Part model, mm, in its own coordinate system. Face numbers are marked on the shaded views. A direction names the side the tool comes from. Round coordinates to 2 decimals unless told otherwise and drop trailing zeros. Loops run counter-clockwise (first coordinate to the right, second up) from the corner with the lowest first, then second, coordinate; pieces in that order, holes last. Notation, with made-up numbers: (50.5, 60) - (78.5, 60) arc R15 ccw to (78.5, 79) - close; hole circle Ø3 at (12, 45.5). An arc over 180 degrees is marked (long way). Put each result on its own line as item: value.
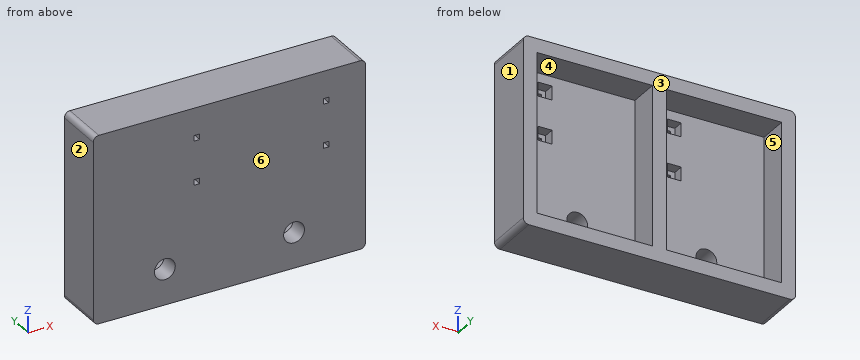
from build123d import *

# Parameters (mm, degrees)
SKETCH1_W           = 65.405
SKETCH1_H           = 85.725
BOSS_EXTRUDE1_DEPTH = 22.86
SKETCH2_W           = 52.705
SKETCH2_H           = 73.025
CUT_EXTRUDE1_DEPTH  = 13.97
SKETCH6_W           = 6.35
SKETCH6_H           = 6.35
CUT_EXTRUDE3_DEPTH  = 5.08
SKETCH7_W           = 2.54
SKETCH7_H           = 2.54
CUT_EXTRUDE4_DEPTH  = 110.496539443
SKETCH5_R           = 4.7625
CUT_EXTRUDE5_DEPTH  = 109.727873841
LPATTERN3_COUNT     = 2
LPATTERN3_PITCH     = 59.055
FILLET1_R           = 2.54


with BuildPart() as part:
    # Sketch1 → Boss-Extrude1 (new body)
    with BuildSketch(Plane(origin=(0, 0, 0), x_dir=(1, 0, 0), z_dir=(0, 1, 0))):
        with Locations((32.7025, 42.8625)):
            Rectangle(SKETCH1_W, SKETCH1_H)
    boss_extrude1 = extrude(amount=BOSS_EXTRUDE1_DEPTH)

    # Sketch2 → Cut-Extrude1 (cut)
    with BuildSketch(Plane(origin=(0, 22.86, 0), x_dir=(1, 0, 0), z_dir=(0, 1, 0))):
        with Locations((32.7025, 42.8625)):
            Rectangle(SKETCH2_W, SKETCH2_H)
    cut_extrude1 = extrude(amount=-CUT_EXTRUDE1_DEPTH, mode=Mode.SUBTRACT)

    # Sketch6 → Cut-Extrude3 (cut)
    with BuildSketch(Plane(origin=(0, 8.89, 0), x_dir=(1, 0, 0), z_dir=(0, 1, 0))):
        with Locations((47.371, 33.782)):
            Rectangle(SKETCH6_W, SKETCH6_H)
        with Locations((47.371, 13.716)):
            Rectangle(SKETCH6_W, SKETCH6_H)
    cut_extrude3 = extrude(amount=-CUT_EXTRUDE3_DEPTH, mode=Mode.SUBTRACT)

    # Sketch7 → Cut-Extrude4 (cut, through all)
    with BuildSketch(Plane(origin=(0, 3.81, 0), x_dir=(1, 0, 0), z_dir=(0, 1, 0))):
        with Locations((47.371, 33.782)):
            Rectangle(SKETCH7_W, SKETCH7_H)
        with Locations((47.371, 13.716)):
            Rectangle(SKETCH7_W, SKETCH7_H)
    cut_extrude4 = extrude(amount=-CUT_EXTRUDE4_DEPTH, mode=Mode.SUBTRACT)

    # Sketch5 → Cut-Extrude5 (cut, through all)
    with BuildSketch(Plane(origin=(0, 8.89, 0), x_dir=(1, 0, 0), z_dir=(0, 1, 0))):
        with Locations(Location((32.7025, 69.469, 0), (0, 0, 270))):
            Circle(SKETCH5_R)
    cut_extrude5 = extrude(amount=-CUT_EXTRUDE5_DEPTH, mode=Mode.SUBTRACT)

    # LPattern3: Boss-Extrude1, Cut-Extrude1, Cut-Extrude3, Cut-Extrude4, Cut-Extrude5 ×2
    with Locations(*[(i * LPATTERN3_PITCH, 0, 0) for i in range(1, LPATTERN3_COUNT)]):
        add(boss_extrude1)
        add(cut_extrude1, mode=Mode.SUBTRACT)
        add(cut_extrude3, mode=Mode.SUBTRACT)
        add(cut_extrude4, mode=Mode.SUBTRACT)
        add(cut_extrude5, mode=Mode.SUBTRACT)

    # Fillet1
    fillet1_edges = [part.edges().sort_by_distance(p)[0] for p in [
        (0, 11.43, -85.725),
        (0, 11.43, 0),
        (124.46, 11.43, -85.725),
        (124.46, 11.43, 0),
    ]]
    fillet(fillet1_edges, radius=FILLET1_R)


solid = part.part
1. Band-saw the part on B-B (z = -66.5). List the corners of the cut face in (x, y) (3 decimals), plus the area to 3 significant figures.
A:
outline: (0, 0) - (28.979, 0) - (28.979, 8.89) - (6.35, 8.89) - (6.35, 22.86) - (0, 22.86) - close; (36.426, 0) - (88.034, 0) - (88.034, 8.89) - (65.405, 8.89) - (65.405, 22.86) - (59.055, 22.86) - (59.055, 8.89) - (36.426, 8.89) - close; (95.481, 0) - (124.46, 0) - (124.46, 22.86) - (118.11, 22.86) - (118.11, 8.89) - (95.481, 8.89) - close
area: 1,240 mm²
2. Band-saw the part on D-D (z = -41). List the corners of the cut face in (x, y) (3 decimals).
A:
outline: (0, 0) - (124.46, 0) - (124.46, 22.86) - (118.11, 22.86) - (118.11, 8.89) - (65.405, 8.89) - (65.405, 22.86) - (59.055, 22.86) - (59.055, 8.89) - (6.35, 8.89) - (6.35, 22.86) - (0, 22.86) - close
3. Two-plate mould, pull along X, no slides. Class the marked faces 1, 2, 3 and 4: pulls with the +X half, pulls with the -X half, needs draft (parallel to the pull), parting line crosses it, or undercut.
A:
face 1: pulls with the +X half
face 2: pulls with the -X half
face 3: needs draft
face 4: undercut
4. Band-saw the part on A-A (y = 12.25). List the corners of the cut face in (x, z) (3 decimals).
A:
outline: (0, -83.185) arc R2.54 ccw to (2.54, -85.725) - (121.92, -85.725) arc R2.54 ccw to (124.46, -83.185) - (124.46, -2.54) arc R2.54 ccw to (121.92, 0) - (2.54, 0) arc R2.54 ccw to (0, -2.54) - close; hole (6.35, -79.375) - (59.055, -79.375) - (59.055, -6.35) - (6.35, -6.35) - close; hole (65.405, -79.375) - (118.11, -79.375) - (118.11, -6.35) - (65.405, -6.35) - close
5. Tool access for the marked faces 5 and 6: list every direction of +Z, -Z, +X, -X, +Y, -Y with a clear straight run to the whole face (end or side of a thin tool).
A:
face 5: +Y
face 6: +Z, -Z, +X, -X, -Y
6. Band-saw the part on C-C (x = 84). List the corners of the cut face in (y, z) (3 decimals).
A:
outline: (0, -85.725) - (22.86, -85.725) - (22.86, -79.375) - (8.89, -79.375) - (8.89, -6.35) - (22.86, -6.35) - (22.86, 0) - (0, 0) - close
7. Probe line 1 along X through (y, z) = (19.5, -79) (3 decimals); line 2 along Z through (x, y) = (107.5, 13) (3 decimals); line 3 along Y through (x, z) = (68, -58.5). List the from-to ranges inside material, lowest first. Write a range as [from, to].
A:
line 1: x = [0, 6.35], [59.055, 65.405], [118.11, 124.46]
line 2: z = [-85.725, -79.375], [-6.35, 0]
line 3: y = [0, 8.89]
8. Pin check, flat tips, straight feed: P1, Ø5, axis at x = 48, z = -33.5, coming from the +Y side; P2, Ø5, axis at x = 46, z = -12.5, coming from the +Y side. Stop position of each tip, or through.
A:
P1: stops at y = 3.81
P2: stops at y = 8.89
